The model under review builds one solid part; all positions refer to its coordinate system, in mm. A direction names the side the tool comes from. Coordinates: 2 decimals unless noted, no trailing zeros. Loops run counter-clockwise (first coordinate to the right, second up) from the corner with the lowest first, then second, coordinate; pieces in that order, holes last. Notation, with made-up numbers: (42.5, 20) - (96.5, 20) arc R14 ccw to (96.5, 42) - close; hole circle Ø8 at (82, 89.25). An arc over 180 degrees is marked (long way). Answer in a Markdown table with one row per item. Add a question column.
(1) Mouldability with a two-part tool opening along X and no side actions: class faces 5 (the cylindrical face through (76.68, 2.79, -0.74)), 6 (the flat face through (-70, 3, -15)), 7 (the flat face through (-55, 3, -18.5)) as +X half, -X half, draft (parallel to the pull), parting line (faces both ways), or undercut.
(2) For P1, Ø1.6, axis at y = 2.5, z = -16, coming from the -X side; P2, Ø3, axis at y = 2.5, z = -15, coming from the +X side; P3, Ø1.5, axis at x = -12.5, y = 1.5, coming from the -Z side; P4, Ø6, axis at x = 80, z = 0, coming from the -Y side, all flat-tipped, find the tip position at first contact; note any pin that passes through.
(3) For line 1 along X through (y, z) = (4.4, 0); line 2 along X through (y, z) = (0.3, -14.5); line 3 along Z through (x, y) = (15, 2.9), list the stretches that pass through material, from the lowest coordinate up.
(4) We need section B-B on z = 0. Write out the cut boundary in (x, y).
(5) We need section C-C on x = 80. Write out the cut boundary in (y, z), plus the area to 3 significant figures.
(6) We need section D-D on x = 38. Write out the cut boundary in (y, z).
(7) We need section A-A on y = 2.35. Write out the cut boundary in (x, z).
(8) Machinability: for faces 1 (the flat face through (-90, 3, -12.5)), 2 (the flat face through (-1, 3, -12.5)), 3 (the flat face through (-2, 3, 12.5)), 4 (the flat face through (70, 3, -15)), which of the approach directions +Z, -Z, +X, -X, +Y, -Y give a long, thin tool a straight path to every point of the face, cutting with its end or side? Answer none if there is none.
from build123d import *

# Parameters (mm, degrees)
SKETCH1_W           = 30
SKETCH1_H           = 6
SKETCH1_W_2         = 220
SKETCH1_H_2         = 25
BOSS_EXTRUDE1_DEPTH = 5.5
SKETCH3_R           = 3.4
CUT_EXTRUDE1_DEPTH  = 112.680347421


with BuildPart() as part:
    # Sketch1 → Boss-Extrude1 (new body)
    with BuildSketch(Plane(origin=(0, 0, 0), x_dir=(1, 0, 0), z_dir=(0, 1, 0))):
        with Locations((-55, 15.5)):
            Rectangle(SKETCH1_W, SKETCH1_H)
        Rectangle(SKETCH1_W_2, SKETCH1_H_2)
        with Locations((55, 15.5)):
            Rectangle(SKETCH1_W, SKETCH1_H)
    extrude(amount=BOSS_EXTRUDE1_DEPTH)

    # Sketch3 → Cut-Extrude1 (cut, through all)
    with BuildSketch(Plane(origin=(0, 5.5, 0), x_dir=(1, 0, 0), z_dir=(0, 1, 0))):
        with Locations(Location((80, 0, 0), (0, 0, 270))):
            Circle(SKETCH3_R)
    extrude(amount=-CUT_EXTRUDE1_DEPTH, mode=Mode.SUBTRACT)


solid = part.part
Outcome:
| question | item | result |
|---|---|---|
| 1 | face 5 | undercut |
| 1 | face 6 | -X half |
| 1 | face 7 | draft |
| 2 | P1 | x = -70 |
| 2 | P2 | x = 70 |
| 2 | P3 | z = -12.5 |
| 2 | P4 | through |
| 3 | line 1 | -110 to 76.6, 83.4 to 110 |
| 3 | line 2 | -70 to -40, 40 to 70 |
| 3 | line 3 | -12.5 to 12.5 |
| 4 | outline | (-110, 0) - (76.6, 0) - (76.6, 5.5) - (-110, 5.5) - close; (83.4, 0) - (110, 0) - (110, 5.5) - (83.4, 5.5) - close |
| 5 | outline | (0, -12.5) - (5.5, -12.5) - (5.5, -3.4) - (0, -3.4) - close; (0, 3.4) - (5.5, 3.4) - (5.5, 12.5) - (0, 12.5) - close |
| 5 | area | 100 mm² |
| 6 | outline | (0, -12.5) - (5.5, -12.5) - (5.5, 12.5) - (0, 12.5) - close |
| 7 | outline | (-110, -12.5) - (-70, -12.5) - (-70, -18.5) - (-40, -18.5) - (-40, -12.5) - (40, -12.5) - (40, -18.5) - (70, -18.5) - (70, -12.5) - (110, -12.5) - (110, 12.5) - (-110, 12.5) - close; hole circle Ø6.8 at (80, 0) |
| 8 | face 1 | -Z, -X, +Y, -Y |
| 8 | face 2 | -Z, +Y, -Y |
| 8 | face 3 | +Z, +X, -X, +Y, -Y |
| 8 | face 4 | -Z, +X, +Y, -Y |
